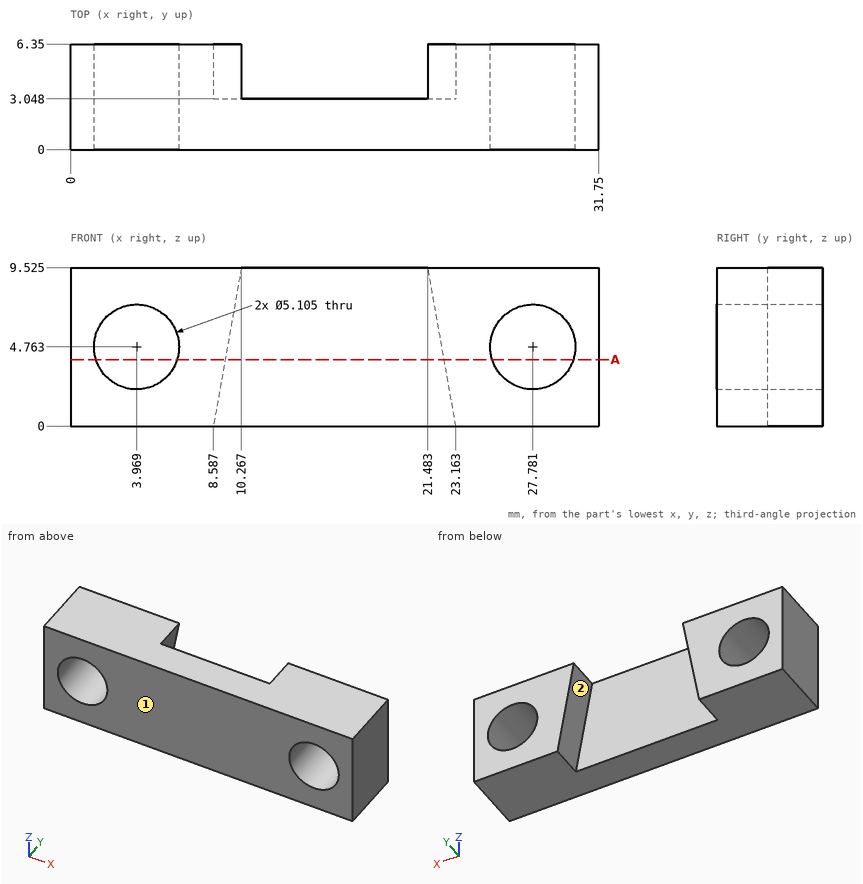
For this review, use the dimensioned drawing (mm, ordinates from the lowest corner) and the shaded views. A direction names the side the tool comes from. Round coordinates to 2 decimals unless told otherwise and drop trailing zeros. Use a Markdown table: item, result.
1) Wall thickness on line 1 along Y through (x, z) = (21.5, 1.25); line 2 along X through (y, z) = (3, 4.5); line 3 along Z through (x, y) = (6, 2) (1 decimal): over which ranges is each line inside the solid? List them lowest first. Write a range as [from, to].
Report:
| item | result |
|---|---|
| line 1 | [0, 3.05] |
| line 2 | [0, 1.43], [6.51, 25.24], [30.32, 31.75] |
| line 3 | [0, 3.2], [6.3, 9.5] |
2) Consider section A-A (z = 4). Give the number of separate pieces and of enclosed holes in the cut face.
Report:
| item | result |
|---|---|
| separate pieces | 3 |
| enclosed holes | 0 |
3) Insertion check: pin 1 (1.5 mm diameter, centred on x = 12.5, y = 4, fed in from +Z); pin 2 (1.5 mm diameter, centred on x = 13.5, y = 3.5, fed in from -Z). Each pin has a flat end and moves straight along its axis. Give the tip position at first contact, or say it passes through.
Report:
| item | result |
|---|---|
| pin 1 | through |
| pin 2 | z = 0 |
4) Tool access review of the marked faces 1 and 2: name each direction out of +Z, -Z, +X, -X, +Y, -Y from which nothing blocks a thin tool from reaching the whole face with its end or side.
Report:
| item | result |
|---|---|
| face 1 | +Z, -Z, +X, -X, -Y |
| face 2 | -Z, +Y |
